Can you work these out from the drawing? Everything is in mm from the part's minimum corner. A direction names the side the tool comes from. Round coordinates to 2 decimals unless told otherwise and drop trailing zeros. Loops run counter-clockwise (first coordinate to the right, second up) from the corner with the lowest first, then second, coordinate; pieces in that order, holes last. Notation, with made-up numbers: M 69,-7.75 L 123,-7.75 A18 ccw 123,7.25 Z; hole C 48.25,-23.75 d9. An arc over 180 degrees is marked long. Answer in a Markdown table with one row per item.
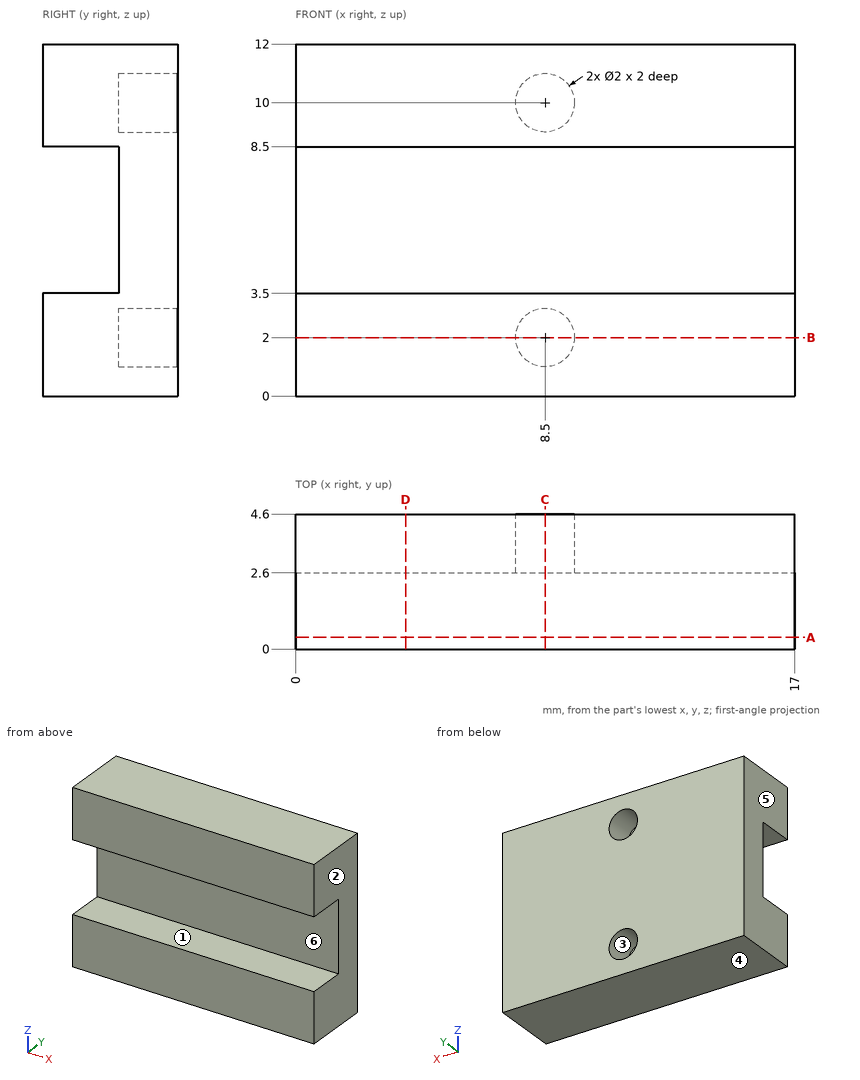
1) I want a section at A-A, the plane y = 0.4. Please give me the cut outline in (x, z).
Computed:
| item | result |
|---|---|
| outline | M 0,0 L 17,0 L 17,3.5 L 0,3.5 Z; M 0,8.5 L 17,8.5 L 17,12 L 0,12 Z |
2) I want a section at B-B, the plane z = 2. Please give me the cut outline in (x, y).
Computed:
| item | result |
|---|---|
| outline | M 0,0 L 17,0 L 17,4.6 L 9.5,4.6 L 9.5,2.6 L 7.5,2.6 L 7.5,4.6 L 0,4.6 Z |
3) I want a section at C-C, the plane x = 8.5. Please give me the cut outline in (y, z), plus the area to 3 significant figures.
Computed:
| item | result |
|---|---|
| outline | M 0,0 L 4.6,0 L 4.6,1 L 2.6,1 L 2.6,3 L 4.6,3 L 4.6,9 L 2.6,9 L 2.6,11 L 4.6,11 L 4.6,12 L 0,12 L 0,8.5 L 2.6,8.5 L 2.6,3.5 L 0,3.5 Z |
| area | 34.2 mm² |
4) I need wall thicknesses on line 1 (Z direction, x = 8.5, y = 3.8); line 2 (Z direction, x = 11.75, y = 1.9); line 3 (Y direction, x = 5.5, z = 7.75). Which ranges of each line are inside material? Lowest first, please.
Computed:
| item | result |
|---|---|
| line 1 | z = 0 to 1, 3 to 9, 11 to 12 |
| line 2 | z = 0 to 3.5, 8.5 to 12 |
| line 3 | y = 2.6 to 4.6 |
5) I want a section at D-D, the plane x = 3.75. Please give me the cut outline in (y, z), plus the area to 3 significant figures.
Computed:
| item | result |
|---|---|
| outline | M 0,0 L 4.6,0 L 4.6,12 L 0,12 L 0,8.5 L 2.6,8.5 L 2.6,3.5 L 0,3.5 Z |
| area | 42.2 mm² |
6) Will these pins go through, and if not, where does the flat tip stop? P1, Ø1.6, axis at x = 8.5, z = 2, coming from the -Y side; P2, Ø1.5, axis at x = 12, z = 6, coming from the -Y side; P3, Ø0.6, axis at x = 8, z = 2, coming from the +Y side.
Computed:
| item | result |
|---|---|
| P1 | stops at y = 0 |
| P2 | stops at y = 2.6 |
| P3 | stops at y = 2.6 |
7) Which directions (+Z, -Z, +X, -X, +Y, -Y) give clear straight access to the entire face, cutting with the end or side of a thin tool? Please do the marked faces 1, 2 and 3.
Computed:
| item | result |
|---|---|
| face 1 | +X, -X, -Y |
| face 2 | +Z, -Z, +X, +Y, -Y |
| face 3 | +Y |
8) If we mould it in two halves opening along Z, with no side actions, what happens to the marked faces 4, 5 and 6? For each: released by +Z, released by -Z, zero draft, split by the parting line, or undercut.
Computed:
| item | result |
|---|---|
| face 4 | released by -Z |
| face 5 | zero draft |
| face 6 | undercut |
